```python
from build123d import *

# Parameters (mm, degrees)
SKETCH_R    = 5
SKETCH_R_2  = 4.2
PAD_DEPTH   = 13
FILLET_R    = 0.2
FILLET001_R = 0.2


with BuildPart() as part:
    # Sketch → Pad (new body)
    with BuildSketch(Plane.XY):
        Circle(SKETCH_R)
        Circle(SKETCH_R_2, mode=Mode.SUBTRACT)
    extrude(amount=PAD_DEPTH)

    # Fillet
    fillet_edges = [part.edges().sort_by_distance(p)[0] for p in [
        (-5, 0, 0),
        (-4.2, 0, 0),
    ]]
    fillet(fillet_edges, radius=FILLET_R)

    # Fillet001
    fillet001_edges = [part.edges().sort_by_distance(p)[0] for p in [
        (-5, 0, 13),
        (-4.2, 0, 13),
    ]]
    fillet(fillet001_edges, radius=FILLET001_R)


solid = part.part
```
The listing builds one solid part. Answer for the finished solid, in the listing's coordinates (mm). Give positions to 0.01 mm unless a question says otherwise; leave off trailing zeros. Write each loop counter-clockwise with the first axis right and the second up, starting at its lowest first coordinate (ties: lowest second). Pieces come first, ordered by that corner, then holes. Notation, with made-up numbers: (60, 27) -> (79, 27) arc R23 ccw to (79, 51) -> close; hole circle Ø8 at (20, 8). An arc over 180 degrees is marked (long way). Write item = value, one per line. Start each with the question number.
1) Straight lines are drawn through the part: line 1 along Y through (x, z) = (0, 9); line 2 along X through (y, z) = (-3.25, 6.5). For each, find the intervals that lie inside material, in ascending order.
2) The part is cut by section A-A, the plane y = 0. Determine the outline of the cut face in (x, z).
3) Each of these flat-tipped pins is pushed along its axis until it touches: pin 1 (1 mm diameter, centred on y = 2.5, z = 3.5, fed in from -X); pin 2 (6 mm diameter, centred on y = 2, z = 1.5, fed in from +X); pin 3 (1.5 mm diameter, centred on y = 2.5, z = 8, fed in from -X). Where does it stop, or does it pass through?
4) The part is cut by section C-C, the plane z = 10. Determine the outline of the cut face in (x, y), and give its area (3 significant figures).
Solutions:
q1.line_1 = -5 to -4.2, 4.2 to 5
q1.line_2 = -3.8 to -2.66, 2.66 to 3.8
q2.outline = (-5, 0.2) arc R0.2 ccw to (-4.8, 0) -> (-4.4, 0) arc R0.2 ccw to (-4.2, 0.2) -> (-4.2, 12.8) arc R0.2 ccw to (-4.4, 13) -> (-4.8, 13) arc R0.2 ccw to (-5, 12.8) -> close; (4.2, 0.2) arc R0.2 ccw to (4.4, 0) -> (4.8, 0) arc R0.2 ccw to (5, 0.2) -> (5, 12.8) arc R0.2 ccw to (4.8, 13) -> (4.4, 13) arc R0.2 ccw to (4.2, 12.8) -> close
q3.pin_1 = -4.58
q3.pin_2 = 5
q3.pin_3 = -4.68
q4.outline = circle Ø10 at (0, 0); hole circle Ø8.4 at (0, 0)
q4.area = 23.1 mm²
